Build history of the part. All positions in model axes, mm. A direction names the side the tool comes from. Give positions to 0.01 mm unless a question says otherwise; leave off trailing zeros. Write each loop counter-clockwise with the first axis right and the second up, starting at its lowest first coordinate (ties: lowest second). Pieces come first, ordered by that corner, then holes. Notation, with made-up numbers: M 30.25,-30 L 89.25,-30 A15 ccw 89.25,-14 Z; hole C 20,8 d1. An arc over 180 degrees is marked long. One line per item, written item: value. Start each with the question number.
from build123d import *

# Parameters (mm, degrees)
EXTRUDE_1_DEPTH       = 27.5
SKETCH_3_R            = 0.75
CUT_EXTRUDE_3_DEPTH   = 3
REVOLVE_1_ANGLE       = 135
MIRROR_3_COPY_1_ANGLE = 135
MIRROR_3_COPY_2_ANGLE = 135
SKETCH_2_R            = 1.5
SKETCH_2_W            = 20
SKETCH_2_H            = 16.5
CUT_EXTRUDE_4_DEPTH   = 3


with BuildPart() as part:
    # 草图1 → 凸台-拉伸1 (new, symmetric)
    with BuildSketch(Plane(origin=(0, 0, 0), x_dir=(1, 0, 0), z_dir=(0, 1, 0))):
        Polygon((-16.617647059, 27.284313725), (25.882352941, 27.284313725), (25.882352941, -27.715686275), (22.882352941, -27.715686275), (22.882352941, 24.284313725), (-16.617647059, 24.284313725), align=None)
    extrude(amount=EXTRUDE_1_DEPTH, both=True)

    # 草图3 → 切除-拉伸3 (cut)
    with BuildSketch(Plane(origin=(25.882352941, 0, 0), x_dir=(0, 0, -1), z_dir=(1, 0, 0))):
        with BuildLine():
            ThreePointArc((-19.394463571, 5.743970558), (-21.414171084, 0), (-19.394463571, -5.743970558))
            Line((-19.394463571, -5.743970558), (-18.726093915, -6.48959236))
            ThreePointArc((-18.726093915, -6.48959236), (-12.715686275, -21), (-6.705278634, -6.48959236))
            Line((-6.705278634, -6.48959236), (-6.036908978, -5.743970558))
            ThreePointArc((-6.036908978, -5.743970558), (-4.017201465, 0), (-6.036908978, 5.743970558))
            Line((-6.036908978, 5.743970558), (-6.705278634, 6.48959236))
            ThreePointArc((-6.705278634, 6.48959236), (-12.715686275, 21), (-18.726093915, 6.48959236))
            Line((-18.726093915, 6.48959236), (-19.394463571, 5.743970558))
        make_face()
        with Locations((-4.215686275, -21)):
            Circle(SKETCH_3_R)
        with Locations((-21.215686275, -21)):
            Circle(SKETCH_3_R)
        with Locations((-4.215686275, 21)):
            Circle(SKETCH_3_R)
        with Locations((-21.215686275, 21)):
            Circle(SKETCH_3_R)
    extrude(amount=-CUT_EXTRUDE_3_DEPTH, mode=Mode.SUBTRACT)

    # 草图5 → 旋转1 (revolve)
    with BuildSketch(Plane(origin=(0, 0, 12.715686275), x_dir=(0, -1, 0), z_dir=(0, 0, 1))):
        Polygon((-22, 25.882352941), (-24.5, 32.882352941), (-23.5, 32.882352941), (-21, 25.882352941), align=None)
    revolve_1 = revolve(axis=Axis((32.882352941, 12.5, 12.715686275), (-1, 0, 0)), revolution_arc=REVOLVE_1_ANGLE)

    # 镜向1: 旋转1 across plane
    add(revolve_1.mirror(Plane.ZX))

    # 镜向2: 旋转1 across plane
    add(revolve_1.mirror(Plane.XY.offset(12.715686275)))

    # 镜向3 copy 1 sketch → 镜向3 copy 1 (revolve)
    with BuildSketch(Plane.YX.offset(-12.715686275)):
        Polygon((-22, 25.882352941), (-24.5, 32.882352941), (-23.5, 32.882352941), (-21, 25.882352941), align=None)
    revolve(axis=Axis((32.882352941, -12.5, 12.715686275), (-1, 0, 0)), revolution_arc=MIRROR_3_COPY_1_ANGLE)

    # 镜向3 copy 2 sketch → 镜向3 copy 2 (revolve)
    with BuildSketch(Plane(origin=(0, 0, 12.715686275), x_dir=(0, -1, 0), z_dir=(0, 0, -1))):
        Polygon((-22, -25.882352941), (-24.5, -32.882352941), (-23.5, -32.882352941), (-21, -25.882352941), align=None)
    revolve(axis=Axis((32.882352941, 12.5, 12.715686275), (1, 0, 0)), revolution_arc=MIRROR_3_COPY_2_ANGLE)

    # 草图2 → 切除-拉伸4 (cut)
    with BuildSketch(Plane(origin=(0, 0, -27.284313725), x_dir=(-1, 0, 0), z_dir=(0, 0, -1))):
        with Locations((6.117647059, -3.5)):
            Circle(SKETCH_2_R)
        with Locations((-13.882352941, -3.5)):
            Circle(SKETCH_2_R)
        with Locations((6.617647059, -19.25)):
            Rectangle(SKETCH_2_W, SKETCH_2_H)
    extrude(amount=-CUT_EXTRUDE_4_DEPTH, mode=Mode.SUBTRACT)


solid = part.part
1) Mould opens along Y. For faces 4 (the face through (3.382, -19, -26)), 5 (the face through (-6, -11, -26)), 6 (the face through (24.4, -21.46, 21.81)) say: released by +Y, released by -Y, zero draft, split by the parting line, or undercut.
2) Band-saw the part on B-B (x = 28.5). List the corners of the cut face in (y, z).
3) Band-saw the part on A-A (y = 12.5). List the corners of the cut face in (x, z), then the cut area to 4 significant figures.
4) Drop flat-ended pins along their axis: P1, Ø4, axis at x = 13.88, y = -3.5, coming from the +Z side; P2, Ø19.5, axis at y = -12.5, z = 12.72, coming from the -X side; P3, Ø0.9, axis at y = -20, z = -25.5, coming from the -X side. Give the stop position or say it passes through.
5) Tool access for faces 1 (the face through (24.4, -21.73, 4.38)), 2 (the face through (22.882, 0, 2)), 3 (the face through (29.139, -5.258, 19.958)): list every direction of +Z, -Z, +X, -X, +Y, -Y with a clear straight run to the whole face (end or side of a thin tool).
6) Band-saw the part on C-C (z = -8). List the corners of the cut face in (x, y), then the cut area to 3 significant figures.
7) Probe line 1 along X through (y, z) = (-3, -25); line 2 along Z through (x, y) = (4.5, -20); line 3 along X through (y, z) = (21.5, -2.5). List the from-to ranges inside material, lowest first. Write a range as from..to.
8) Band-saw the part on D-D (x = 19.5). List the corners of the cut face in (y, z), then the cut area to 3 significant figures.
Model answer:
1. face 4: zero draft
1. face 5: released by -Y
1. face 6: undercut
2. outline: M -5.83,6.04 A9.43 cw long -5.83,19.39 L -5.12,20.09 A10.43 ccw long -5.12,5.34 Z; M 5.12,5.34 A10.43 ccw long 5.12,20.09 L 5.83,19.39 A9.43 cw long 5.83,6.04 Z
3. outline: M -16.62,-27.28 L 25.88,-27.28 L 25.88,3.22 L 32.88,0.72 L 32.88,1.72 L 25.88,4.22 L 22.88,4.22 L 22.88,-24.28 L -16.62,-24.28 Z; M 22.88,21.22 L 25.88,21.22 L 32.88,23.72 L 32.88,24.72 L 25.88,22.22 L 25.88,27.72 L 22.88,27.72 Z
3. area: 246.5 mm²
4. P1: stops at z = -24.28
4. P2: stops at x = 22.88
4. P3: stops at x = 3.38
5. face 1: -X
5. face 2: +Z, -X, +Y, -Y
5. face 3: +X
6. outline: M 22.88,-27.5 L 25.88,-27.5 L 25.88,27.5 L 22.88,27.5 Z
6. area: 165 mm²
7. line 1: x = -16.62..-7.53, -4.7..12.47, 15.3..25.88
7. line 2: z = -27.28..-24.28
7. line 3: x = 22.88..25.88
8. outline: M -27.5,-27.28 L 27.5,-27.28 L 27.5,-24.28 L -27.5,-24.28 Z
8. area: 165 mm²
